Geometry check sheet. Reference: the model listing, model coordinates, mm. Face numbers are marked on the shaded views. A direction names the side the tool comes from. Coordinates: 2 decimals unless noted, no trailing zeros. Write each loop counter-clockwise with the first axis right and the second up, starting at its lowest first coordinate (ties: lowest second). Pieces come first, ordered by that corner, then holes. Notation, with made-up numbers: (76.5, 58.5) -> (113.5, 58.5) arc R27 ccw to (113.5, 77.5) -> close; hole circle Ø7 at (65, 25). An arc over 180 degrees is marked (long way). Use a Markdown table: item, result.
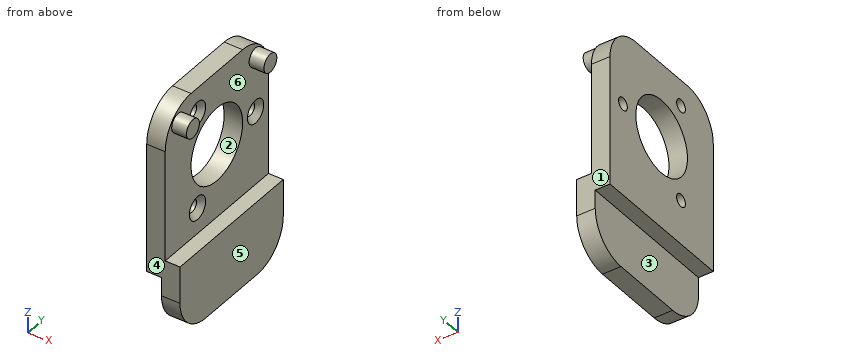
```python
from build123d import *

# Parameters (mm, degrees)
SKETCH1_R                                       = 10
BOSS_EXTRUDE1_DEPTH                             = 5
CSK_FOR_M3_FLAT_HEAD_MACHINE_SCREW1_D           = 3.4
CSK_FOR_M3_FLAT_HEAD_MACHINE_SCREW1_CSINK_D     = 6.3
CSK_FOR_M3_FLAT_HEAD_MACHINE_SCREW1_CSINK_ANGLE = 90
SKETCH4_W                                       = 5
SKETCH4_H                                       = 40
BOSS_EXTRUDE2_DEPTH                             = 9
SKETCH5_W                                       = 5
SKETCH5_H                                       = 40
BOSS_EXTRUDE3_DEPTH                             = 15
FILLET2_R                                       = 10
SKETCH6_R                                       = 2.5
BOSS_EXTRUDE4_DEPTH                             = 4


with BuildPart() as part:
    # Sketch1 → Boss-Extrude1 (new body)
    with BuildSketch(Plane(origin=(0, 0, 0), x_dir=(0, 0, -1), z_dir=(1, 0, 0))):
        with BuildLine():
            Line((10, 20), (20, 20))
            Line((20, 20), (20, 10))
            Line((20, 10), (20, -10))
            Line((20, -10), (20, -20))
            Line((20, -20), (10, -20))
            Line((10, -20), (-10, -20))
            ThreePointArc((-10, -20), (-17.071067812, -17.071067812), (-20, -10))
            Line((-20, -10), (-20, 10))
            ThreePointArc((-20, 10), (-17.071067812, 17.071067812), (-10, 20))
            Line((-10, 20), (10, 20))
        make_face()
        Circle(SKETCH1_R, mode=Mode.SUBTRACT)
    extrude(amount=BOSS_EXTRUDE1_DEPTH)

    # CSK for M3 Flat Head Machine Screw1 (through all)
    with Locations(Plane(origin=(5, 0, 0), x_dir=(0, 0, -1), z_dir=(1, 0, 0))):
        with Locations((0, 15), (12.990381057, -7.5), (-12.990381057, -7.5)):
            CounterSinkHole(CSK_FOR_M3_FLAT_HEAD_MACHINE_SCREW1_D / 2, CSK_FOR_M3_FLAT_HEAD_MACHINE_SCREW1_CSINK_D / 2, counter_sink_angle=CSK_FOR_M3_FLAT_HEAD_MACHINE_SCREW1_CSINK_ANGLE)

    # Sketch4 → Boss-Extrude2 (add)
    with BuildSketch(Plane.ZY):
        with Locations((-22.5, 0)):
            Rectangle(SKETCH4_W, SKETCH4_H)
    extrude(amount=-BOSS_EXTRUDE2_DEPTH)

    # Sketch5 → Boss-Extrude3 (add)
    with BuildSketch(Plane(origin=(0, 0, -25), x_dir=(-1, 0, 0), z_dir=(0, 0, -1))):
        with Locations((-6.5, 0)):
            Rectangle(SKETCH5_W, SKETCH5_H)
    extrude(amount=BOSS_EXTRUDE3_DEPTH)

    # Fillet2
    fillet2_edges = [part.edges().sort_by_distance(p)[0] for p in [
        (6.5, 20, -40),
        (6.5, -20, -40),
    ]]
    fillet(fillet2_edges, radius=FILLET2_R)

    # Sketch6 → Boss-Extrude4 (add)
    with BuildSketch(Plane(origin=(5, 0, 0), x_dir=(0, 0, -1), z_dir=(1, 0, 0))):
        with Locations((-15, -15)):
            Circle(SKETCH6_R)
        with Locations((-15, 15)):
            Circle(SKETCH6_R)
    extrude(amount=BOSS_EXTRUDE4_DEPTH)


solid = part.part
```
Item 1: Section check A-A on z = 0. Record the boundary of the cut face in (x, y), then the cut area to 3 significant figures.
Answer block:
| item | result |
|---|---|
| outline | (0, -20) -> (5, -20) -> (5, -10) -> (0, -10) -> close; (0, 10) -> (5, 10) -> (5, 11.85) -> (3.55, 13.3) -> (0, 13.3) -> close; (0, 16.7) -> (3.55, 16.7) -> (5, 18.15) -> (5, 20) -> (0, 20) -> close |
| area | 80.9 mm^2 |
Item 2: Section check D-D on z = -9. Record the boundary of the cut face in (x, y), then the cut area to 3 significant figures.
Answer block:
| item | result |
|---|---|
| outline | (0, -20) -> (5, -20) -> (5, -4.36) -> (0, -4.36) -> close; (0, 4.36) -> (5, 4.36) -> (5, 20) -> (0, 20) -> close |
| area | 156 mm^2 |
Item 3: Tool access check on the marked faces 5 and 6. Record the directions out of +Z, -Z, +X, -X, +Y, -Y that give a thin tool (end or side, any length) a straight path to the whole face; none if there is none.
Answer block:
| item | result |
|---|---|
| face 5 | +Z, -Z, +X, +Y, -Y |
| face 6 | +X |
Item 4: Depth check by flat-ended pin: P1, Ø7.5, axis at y = 1, z = -32, coming from the -X side; P2, Ø20, axis at y = 6, z = -7, coming from the +X side; P3, Ø5.5, axis at y = -7.5, z = -12.99, coming from the +X side. Enter the tip coordinate at first touch or a pass-through.
Answer block:
| item | result |
|---|---|
| P1 | stops at x = 4 |
| P2 | stops at x = 5 |
| P3 | stops at x = 4.6 |
Item 5: Section check B-B on y = 0. Record the boundary of the cut face in (x, z).
Answer block:
| item | result |
|---|---|
| outline | (0, -25) -> (4, -25) -> (4, -40) -> (9, -40) -> (9, -20) -> (5, -20) -> (5, -10) -> (0, -10) -> close; (0, 10) -> (5, 10) -> (5, 20) -> (0, 20) -> close |
Item 6: Mould release check, pull along Y, two halves, no side actions. Record for the marked faces 1, 2, 3 and 4: +Y half, -Y half, draft (parallel to the pull), parting line (faces both ways), or undercut.
Answer block:
| item | result |
|---|---|
| face 1 | +Y half |
| face 2 | undercut |
| face 3 | draft |
| face 4 | -Y half |
Item 7: Section check C-C on y = -7.5. Record the boundary of the cut face in (x, z), then the cut area to 3 significant figures.
Answer block:
| item | result |
|---|---|
| outline | (0, -25) -> (4, -25) -> (4, -40) -> (9, -40) -> (9, -20) -> (5, -20) -> (5, -16.14) -> (3.55, -14.69) -> (0, -14.69) -> close; (0, -11.29) -> (3.55, -11.29) -> (5, -9.84) -> (5, -6.61) -> (0, -6.61) -> close; (0, 6.61) -> (5, 6.61) -> (5, 9.84) -> (3.55, 11.29) -> (0, 11.29) -> close; (0, 14.69) -> (3.55, 14.69) -> (5, 16.14) -> (5, 20) -> (0, 20) -> close |
| area | 216 mm^2 |
Item 8: Thickness scan on L1, parallel to Y at x = 1.85, z = 0; L2, parallel to Z at x = 0.8, y = -7.5; L3, parallel to Y at x = 4.5, z = 0. Record the ranges inside material, lowest first. Write a range as [from, to].
Answer block:
| item | result |
|---|---|
| L1 | y = [-20, -10], [10, 13.3], [16.7, 20] |
| L2 | z = [-25, -14.69], [-11.29, -6.61], [6.61, 11.29], [14.69, 20] |
| L3 | y = [-20, -10], [10, 12.35], [17.65, 20] |
